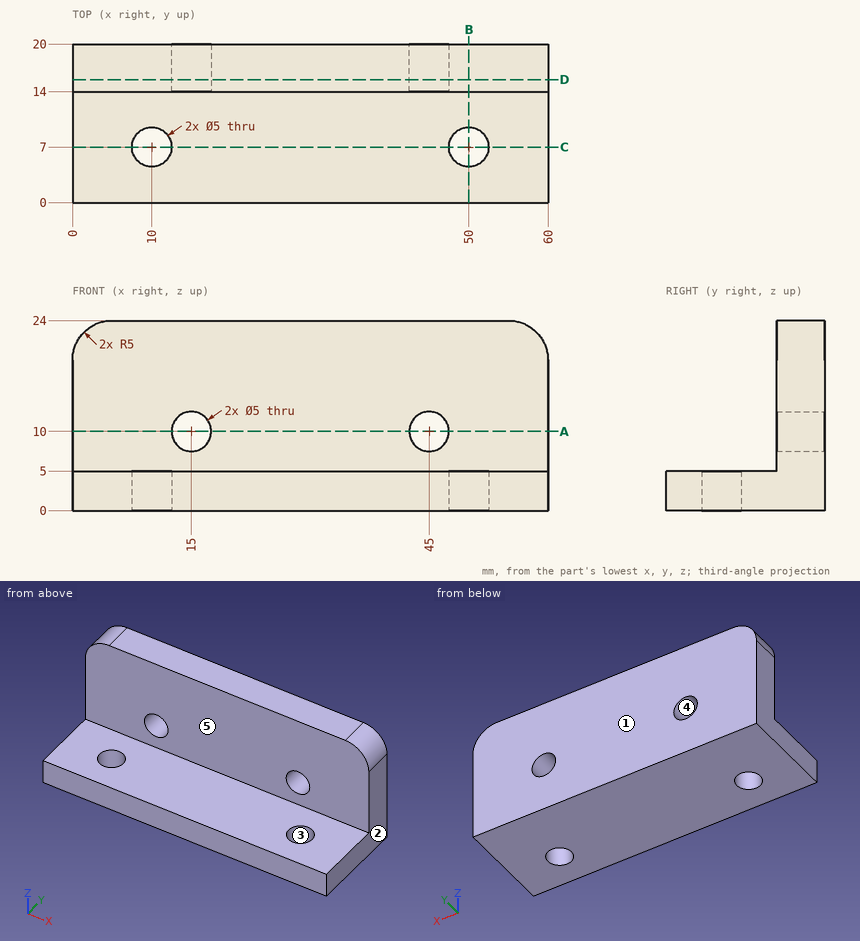
Could you check a few things on this drawing? It's one solid part, dimensions in mm from its lowest x, y, z. A direction names the side the tool comes from. Give positions to 0.01 mm unless a question says otherwise; leave off trailing zeros. Write each loop counter-clockwise with the first axis right and the second up, starting at its lowest first coordinate (ties: lowest second). Pieces come first, ordered by that corner, then holes. Notation, with made-up numbers: (65, -32) - (99, -32) arc R19 cw to (99, -4) - close; hole circle Ø3 at (74.5, 24.25). An arc over 180 degrees is marked (long way). Use CSV: the item, a comma, the result in double quotes. Start each with the question number.
Item 1: For the marked faces 4 and 5, which set-ups out of +Z, -Z, +X, -X, +Y, -Y let a thin tool reach every point of the face, with its end or its side?
Item 2: I'm going to push flat-ended pins straight in: pin 1 (8 mm diameter, centred on x = 15, z = 10, fed in from -Y); pin 2 (3 mm diameter, centred on x = 33, y = 8, fed in from +Z); pin 3 (10 mm diameter, centred on y = 5.5, z = 17.5, fed in from +X). Where does each tip first touch, or does it pass through?
Item 3: If we mould it in two halves opening along Y, with no side actions, what happens to the marked faces 1, 2 and 3? For each: pulls with the +Y half, pulls with the -Y half, needs draft (parallel to the pull), parting line crosses it, or undercut.
Item 4: I want a section at C-C, the plane y = 7. Please give me the cut outline in (x, z), then the cut area to 3 significant figures.
Item 5: I want a section at A-A, the plane z = 10. Please give me the cut outline in (x, y), then the cut area to 3 significant figures.
Item 6: I want a section at D-D, the plane y = 15.5. Please give me the cut outline in (x, z), then the cut area to 3 significant figures.
Item 7: I want a section at B-B, the plane x = 50. Please give me the cut outline in (y, z).
Item 8: If I drill on line 1 along Z through (x, y) = (15, 17.85); line 2 along Y through (x, z) = (23.5, 16.5); line 3 along Z through (x, y) = (5, 5), over which ranges is the centre line in solid material (lowest first)?
Findings:
1,face 4,"+Y, -Y"
1,face 5,"+Z, +X, -X, -Y"
2,pin 1,"stops at y = 14"
2,pin 2,"stops at z = 5"
2,pin 3,"passes through"
3,face 1,"pulls with the +Y half"
3,face 2,"needs draft"
3,face 3,"undercut"
4,outline,"(0, 0) - (7.5, 0) - (7.5, 5) - (0, 5) - close; (12.5, 0) - (47.5, 0) - (47.5, 5) - (12.5, 5) - close; (52.5, 0) - (60, 0) - (60, 5) - (52.5, 5) - close"
4,area,"250 mm2"
5,outline,"(0, 14) - (12.5, 14) - (12.5, 20) - (0, 20) - close; (17.5, 14) - (42.5, 14) - (42.5, 20) - (17.5, 20) - close; (47.5, 14) - (60, 14) - (60, 20) - (47.5, 20) - close"
5,area,"300 mm2"
6,outline,"(0, 0) - (60, 0) - (60, 19) arc R5 ccw to (55, 24) - (5, 24) arc R5 ccw to (0, 19) - close; hole circle Ø5 at (15, 10); hole circle Ø5 at (45, 10)"
6,area,"1,390 mm2"
7,outline,"(0, 0) - (4.5, 0) - (4.5, 5) - (0, 5) - close; (9.5, 0) - (20, 0) - (20, 24) - (14, 24) - (14, 5) - (9.5, 5) - close"
8,line 1,"z = 0 to 7.5, 12.5 to 24"
8,line 2,"y = 14 to 20"
8,line 3,"z = 0 to 5"
